Verification items for the finished model (mm, model axes). A direction names the side the tool comes from. Give positions to 0.01 mm unless a question says otherwise; leave off trailing zeros. Write each loop counter-clockwise with the first axis right and the second up, starting at its lowest first coordinate (ties: lowest second). Pieces come first, ordered by that corner, then holes. Notation, with made-up numbers: (52.25, 58) - (86.25, 58) arc R17 ccw to (86.25, 84) - close; hole circle Ø8 at (-3, 7.5). An arc over 180 degrees is marked (long way). Answer as a JSON object with one key per item and string values. Group by question number.
Item 1: Tool access check on faces 4 (the face through (-25, -1.6, 55.1)), 5 (the face through (-13, -14, 75)), 6 (the face through (-19.417, 22.495, 34.505)), 7 (the face through (-19.417, -22.495, 35.495)), 8 (the face through (-14, 21, 88)). Record the directions out of +Z, -Z, +X, -X, +Y, -Y that give a thin tool (end or side, any length) a straight path to the whole face; none if there is none.
Item 2: Sectioned sample at C-C, the plane z = 74. Record the boundary of the cut face in (x, y).
Item 3: Sectioned sample at A-A, the plane z = 35. Record the boundary of the cut face in (x, y).
Item 4: Sectioned sample at D-D, the plane z = 47. Record the boundary of the cut face in (x, y).
Item 5: Sectioned sample at B-B, the plane x = 0. Record the boundary of the cut face in (y, z), and give its area (3 significant figures).
Item 6: Scan lines: line 1 along Y through (x, z) = (14, 35); line 2 along Y through (x, z) = (-7.5, 35); line 3 along Z through (x, y) = (4.5, -13.5). Record each from-to range of solid material in increasing order. Write a range as [from, to].
Item 7: Go/stop test with flat-tipped pins: pin 1 (6 mm diameter, centred on x = -3.5, z = 72.5, fed in from +Y) (3 decimals); pin 2 (1.5 mm diameter, centred on x = 10.5, y = -18.5, fed in from -Z); pin 3 (22 mm diameter, centred on x = 2.5, z = 72, fed in from -Y). Record where each tip stops, or that it passes through.
Item 8: Draft check along Y on faces 1 (the face through (0, 0, 60)), 2 (the face through (25, -1.6, 55.1)), 3 (the face through (19.614, -22.495, 35.495)). Enter one of: +Y half, -Y half, draft (parallel to the pull), parting line (faces both ways), or undercut.
```python
from build123d import *

# Parameters (mm, degrees)
SKETCH1_R               = 25
BOSS_EXTRUDE3_DEPTH     = 100
SKETCH4_R               = 22.5
BOSS_EXTRUDE4_DEPTH     = 25
SKETCH5_R               = 20
CUT_EXTRUDE2_DEPTH      = 50
CHAMFER1_SIZE           = 5
SKETCH9_W               = 10
SKETCH9_H               = 60.112874217
CUT_EXTRUDE3_DEPTH      = 26.0000001
CUT_EXTRUDE3_DEPTH_BACK = 26.0000001
CUT_EXTRUDE4_DEPTH      = 30
SKETCH12_R              = 26
SKETCH12_R_2            = 25
BOSS_EXTRUDE6_DEPTH     = 2


with BuildPart() as part:
    # Sketch1 → Boss-Extrude3 (new body)
    with BuildSketch(Plane.XY):
        Circle(SKETCH1_R)
    extrude(amount=BOSS_EXTRUDE3_DEPTH)

    # Sketch4 → Boss-Extrude4 (add, symmetric)
    with BuildSketch(Plane(origin=(0, 0, 0), x_dir=(0, 0, -1), z_dir=(1, 0, 0))):
        with Locations((-35, 0)):
            Circle(SKETCH4_R)
    extrude(amount=BOSS_EXTRUDE4_DEPTH, both=True)

    # Sketch5 → Cut-Extrude2 (cut)
    with BuildSketch(Plane(origin=(25, 0, 0), x_dir=(0, 0, -1), z_dir=(1, 0, 0))):
        with Locations((-35, 0)):
            Circle(SKETCH5_R)
    extrude(amount=-CUT_EXTRUDE2_DEPTH, mode=Mode.SUBTRACT)

    # Chamfer1
    chamfer1_edges = [part.edges().sort_by_distance(p)[0] for p in [
        (-25, 0, 0),
    ]]
    chamfer(chamfer1_edges, length=CHAMFER1_SIZE)

    # Sketch9 → Cut-Extrude3 (cut, two sides)
    with BuildSketch(Plane(origin=(0, 0, 0), x_dir=(0, 0, -1), z_dir=(1, 0, 0))) as cut_extrude3_sk:
        with Locations((-95, -5.056437109)):
            Rectangle(SKETCH9_W, SKETCH9_H)
    extrude(amount=CUT_EXTRUDE3_DEPTH, mode=Mode.SUBTRACT)
    extrude(cut_extrude3_sk.sketch, amount=-CUT_EXTRUDE3_DEPTH_BACK, mode=Mode.SUBTRACT)

    # Sketch11 → Cut-Extrude4 (cut)
    with BuildSketch(Plane.XY.offset(90)):
        with BuildLine():
            Line((-10, 15), (10, 15))
            ThreePointArc((10, 15), (13.535533906, 13.535533906), (15, 10))
            Line((15, 10), (15, -10))
            ThreePointArc((15, -10), (13.535533906, -13.535533906), (10, -15))
            Line((10, -15), (-10, -15))
            ThreePointArc((-10, -15), (-13.535533906, -13.535533906), (-15, -10))
            Line((-15, -10), (-15, 10))
            ThreePointArc((-15, 10), (-13.535533906, 13.535533906), (-10, 15))
        make_face()
    extrude(amount=-CUT_EXTRUDE4_DEPTH, mode=Mode.SUBTRACT)

    # Sketch12 → Boss-Extrude6 (add)
    with BuildSketch(Plane.XY.offset(90)):
        Circle(SKETCH12_R)
        Circle(SKETCH12_R_2, mode=Mode.SUBTRACT)
    extrude(amount=-BOSS_EXTRUDE6_DEPTH)


solid = part.part
```
Geometry check:
{
 "1": {"face 4": "-Z, -X, +Y, -Y", "face 5": "+Z", "face 6": "-X, +Y", "face 7": "-X, -Y", "face 8": "none"},
 "2": {"outline": "circle Ø50 at (0, 0); hole (-15, -10) arc R5 ccw to (-10, -15) - (10, -15) arc R5 ccw to (15, -10) - (15, 10) arc R5 ccw to (10, 15) - (-10, 15) arc R5 ccw to (-15, 10) - close"},
 "3": {"outline": "(-25, -22.5) - (-10.9, -22.5) arc R25 ccw to (10.9, -22.5) - (25, -22.5) - (25, -20) - (-25, -20) - close; (-25, 20) - (25, 20) - (25, 22.5) - (10.9, 22.5) arc R25 ccw to (-10.9, 22.5) - (-25, 22.5) - close"},
 "4": {"outline": "(-25, -19.03) - (-16.21, -19.03) arc R25 ccw to (16.21, -19.03) - (25, -19.03) - (25, -16) - (-25, -16) - close; (-25, 16) - (25, 16) - (25, 19.03) - (16.21, 19.03) arc R25 ccw to (-16.21, 19.03) - (-25, 19.03) - close"},
 "5": {"outline": "(-26, 88) - (-25, 88) - (-25, 5) - (-20, 0) - (20, 0) - (25, 5) - (25, 88) - (26, 88) - (26, 90) - (15, 90) - (15, 60) - (-15, 60) - (-15, 90) - (-26, 90) - close; hole circle Ø40 at (0, 35)", "area": "2,320 mm^2"},
 "6": {"line 1": "[-22.5, -20], [20, 22.5]", "line 2": "[-23.85, -20], [20, 23.85]", "line 3": "[0, 20.24], [49.76, 60]"},
 "7": {"pin 1": "y = 24.995", "pin 2": "z = 0.52", "pin 3": "y = -25"},
 "8": {"face 1": "undercut", "face 2": "draft", "face 3": "-Y half"}
}
